from build123d import *

# Parameters (mm, degrees)
F1_DEPTH = 300
F3_DEPTH = 1400


with BuildPart() as f1:
    # F0 (on Front) → F1 (new body)
    with BuildSketch(Plane.XZ):
        Polygon((0, 0), (15, 0), (15, 541.767756), (15, 556.767756), (15, 891.767756), (15, 906.767756), (15, 1241.767756), (15, 1256.767756), (15, 1591.767756), (15, 1606.767756), (15, 1941.767756), (15, 1956.767756), (15, 2500), (1507.518325, 1956.767756), (1548.730486, 1941.767756), (1554.054528, 1955.792629), (0, 2521.42222), align=None)
        Polygon((15, 556.767756), (15, 541.767756), (1304.550659, 541.767756), (1307.166871, 556.767756), align=None)
        Polygon((15, 906.767756), (15, 891.767756), (1365.595615, 891.767756), (1368.211828, 906.767756), align=None)
        Polygon((15, 1941.767756), (1548.730486, 1941.767756), (1507.518325, 1956.767756), (15, 1956.767756), align=None)
        Polygon((15, 1256.767756), (15, 1241.767756), (1426.640572, 1241.767756), (1429.256785, 1256.767756), align=None)
        Polygon((1490.301742, 1606.767756), (15, 1606.767756), (15, 1591.767756), (1487.685529, 1591.767756), align=None)
    extrude(amount=F1_DEPTH)

    # F2 (on face) → F3 (join)
    with BuildSketch(Plane.YZ.offset(15)):
        Polygon((-91.845083, 116.005562), (-300, 191.767756), (-300, 0), (-285, 0), (-285, 170.345536), (-82.879996, 96.77987), (0, 324.490787), (0, 368.347853), align=None)
    extrude(amount=F3_DEPTH)


solid = f1.part
Can you work these out from the model? Positions are in its coordinate system, mm. A direction names the side the tool comes from. Give positions to 0.01 mm unless a question says otherwise; leave off trailing zeros. Loops run counter-clockwise (first coordinate to the right, second up) from the corner with the lowest first, then second, coordinate; pieces in that order, holes last. Notation, with made-up numbers: (17, 21) -> (57, 21) arc R27 ccw to (57, 50) -> close; hole circle Ø10 at (-1, 59). An arc over 180 degrees is marked (long way). Return JSON: item names as keys, results as strings.
Q1. For pin 1 Ø12 at (x, y) = (1092.5, -266) entering from +Z; pin 2 Ø10 at (x, y) = (746, -147) entering from -Z; pin 3 Ø3 at (y, z) = (-223.5, 800) entering from +X, each with a flat end and sliding along its axis, tell me the tip position at first contact or that it passes through.
Checks:
{"pin 1": "stops at z = 2125.97", "pin 2": "stops at z = 118.3", "pin 3": "stops at x = 15"}
Q2. I want a section at B-B, the plane z = 2358. List the corners of the cut face in (x, y) for me, then the cut area to 3 significant figures.
Checks:
{"outline": "(0, -300) -> (15, -300) -> (15, 0) -> (0, 0) -> close; (405.14, -300) -> (449, -300) -> (449, 0) -> (405.14, 0) -> close", "area": "17,700 mm2"}
Q3. On a 3-axis mill with a long thin cutter (end or side, diameter ignored), from which of +Z, -Z, +X, -X, +Y, -Y can I reach the whole of each face in a straight line? I mean faces 4 (the face through (705.2, -194.47, 153.36)), 5 (the face through (772, -148, 1956.768)), 6 (the face through (711, -148, 1241.768)). Say none if no direction works.
Checks:
{"face 4": "+X", "face 5": "+Y, -Y", "face 6": "+X, +Y, -Y"}
Q4. We'd pull the mould along Y, two halves only. Please class faces 1 (the face through (15, -148, 2225)), 2 (the face through (705.2, -45.28, 243.94)), 3 (the face through (705.2, -42.02, 209.04)): released by +Y, released by -Y, zero draft, split by the parting line, or undercut.
Checks:
{"face 1": "zero draft", "face 2": "undercut", "face 3": "released by +Y"}
Q5. I want a section at A-A, the plane x = 918.5. Count the separate pieces of the cut face and the enclosed holes in it, then the cut area to 3 significant figures.
Checks:
{"separate pieces": "7", "enclosed holes": "0", "area": "37,100 mm2"}
Q6. I need wall thicknesses on probe 1 along Z at (x, y) = (1448, -223.5); probe 2 along X at (y, z) = (-31, 465.5); probe 3 along Z at (x, y) = (1410, -97). Which ranges of each line are inside material? Lowest first, please.
Checks:
{"probe 1": "z = 1591.77 to 1606.77, 1941.77 to 1956.77, 1978.43 to 1994.39", "probe 2": "x = 0 to 15", "probe 3": "z = 101.92 to 117.88, 1241.77 to 1256.77, 1591.77 to 1606.77, 1941.77 to 1956.77, 1992.26 to 2008.22"}
Q7. I want a section at D-D, the plane z = 1211.5. List the corners of the cut face in (x, y) for me, then the cut area to 3 significant figures.
Checks:
{"outline": "(0, -300) -> (15, -300) -> (15, 0) -> (0, 0) -> close", "area": "4,500 mm2"}
